The listing builds one solid part. Answer for the finished solid, in the listing's coordinates (mm). Coordinates: 2 decimals unless noted, no trailing zeros. Loops run counter-clockwise (first coordinate to the right, second up) from the corner with the lowest first, then second, coordinate; pieces in that order, holes last. Notation, with made-up numbers: (32, -4.75) -> (66, -4.75) arc R18 ccw to (66, 24.25) -> close; hole circle Ø2 at (60, 5.5). An arc over 180 degrees is marked (long way). Answer in a Markdown table with one row per item.
```python
from build123d import *

# Parameters (mm, degrees)
F0_W        = 101.6
F0_H        = 101.6
F1_DEPTH    = 166
F2_R        = 3.175
F3_DEPTH    = 101.601
F4_T1_DEPTH = 176


# Not quite as in the source:
# - a fillet or chamfer that OpenCascade refuses, or shapes differently, is made with other operations: its cross-section is extruded or revolved along the edge and cut away or added


with BuildPart() as f1:
    # F0 (on Front) → F1 (new body)
    with BuildSketch(Plane.XZ):
        Rectangle(F0_W, F0_H)
    extrude(amount=F1_DEPTH)

    # F2 (on face) → F3 (cut, through all)
    with BuildSketch(Plane.YZ.offset(50.8)):
        with Locations((-143, 46.3)):
            Circle(F2_R)
        with Locations((-83, 46.3)):
            Circle(F2_R)
        with Locations((-23, 46.3)):
            Circle(F2_R)
    extrude(amount=-F3_DEPTH, mode=Mode.SUBTRACT)

    # F4: fillet of radius 2 on 1 edges, made by hand

    # F4_s2 → F4_t1 (cut)
    with BuildSketch(Plane.XZ.offset(-5)):
        with BuildLine():
            ThreePointArc((50.8, 48.8), (50.2142135624, 50.2142135624), (48.8, 50.8))
            Line((48.8, 50.8), (50.8, 50.8))
            Line((50.8, 50.8), (50.8, 48.8))
        make_face()
    extrude(amount=F4_T1_DEPTH, mode=Mode.SUBTRACT)


solid = f1.part
```
Item 1: A cutting plane is placed at B-B, the plane y = -83. Determine the outline of the cut face in (x, z) (3 decimals), plus the area to 3 significant figures.
Findings below:
| item | result |
|---|---|
| outline | (-50.8, -50.8) -> (50.8, -50.8) -> (50.8, 43.125) -> (-50.8, 43.125) -> close; (-50.8, 49.475) -> (50.683, 49.475) arc R2 ccw to (48.8, 50.8) -> (-50.8, 50.8) -> close |
| area | 9,680 mm2 |
Item 2: Determine the mould class of faces 1 (the face through (-1, -166, 1)), 2 (the face through (-1, 0, 1)), 3 (the face through (0.71, -23.41, 49.45)) for opening direction Y: +Y half, -Y half, draft (parallel to the pull), parting line (faces both ways), or undercut.
Findings below:
| item | result |
|---|---|
| face 1 | -Y half |
| face 2 | +Y half |
| face 3 | undercut |
Item 3: Find the intervals of material crossed by probe 1 along Y at (x, z) = (-14, 46.3) (3 decimals); probe 2 along Z at (x, y) = (1.5, -23) (3 decimals); probe 3 along Y at (x, z) = (17, 44), in increasing order.
Findings below:
| item | result |
|---|---|
| probe 1 | y = -166 to -146.175, -139.825 to -86.175, -79.825 to -26.175, -19.825 to 0 |
| probe 2 | z = -50.8 to 43.125, 49.475 to 50.8 |
| probe 3 | y = -166 to -145.19, -140.81 to -85.19, -80.81 to -25.19, -20.81 to 0 |
Item 4: A cutting plane is placed at A-A, the plane z = 46.3. Determine the outline of the cut face in (x, y) (3 decimals).
Findings below:
| item | result |
|---|---|
| outline | (-50.8, -166) -> (50.8, -166) -> (50.8, -146.175) -> (-50.8, -146.175) -> close; (-50.8, -139.825) -> (50.8, -139.825) -> (50.8, -86.175) -> (-50.8, -86.175) -> close; (-50.8, -79.825) -> (50.8, -79.825) -> (50.8, -26.175) -> (-50.8, -26.175) -> close; (-50.8, -19.825) -> (50.8, -19.825) -> (50.8, 0) -> (-50.8, 0) -> close |
